Read the model definition and answer for the solid it produces. Units are mm, in the model's axes. Coordinates: 2 decimals unless noted, no trailing zeros. Write each loop counter-clockwise with the first axis right and the second up, starting at its lowest first coordinate (ties: lowest second). Pieces come first, ordered by that corner, then holes.
(1) The part is cut by section B-B, the plane z = 2.25. Determine the outline of the cut face in (x, y).
(2) The part is cut by section A-A, the plane y = 3.8. Determine the outline of the cut face in (x, z), and give its area (3 significant figures).
(3) Straight lines are drawn through the part: line 1 along X through (y, z) = (4.6, 2); line 2 along Z through (x, y) = (9, 0.6). For each, find the intervals that lie inside material, in ascending order.
(4) The part is cut by section C-C, the plane x = 10. Determine the outline of the cut face in (y, z), and give its area (3 significant figures).
```python
from build123d import *

# Parameters (mm, degrees)
BOSS_EXTRUDE1_DEPTH = 5


with BuildPart() as part:
    # Sketch1 → Boss-Extrude1 (new body)
    with BuildSketch(Plane(origin=(0, 0, 0), x_dir=(1, 0, 0), z_dir=(0, 1, 0))):
        with BuildLine():
            Line((75, -15), (75, 0))
            Line((75, 0), (14.1, 0))
            ThreePointArc((14.1, 0), (10, -4.1), (5.9, 0))
            Line((5.9, 0), (0, 0))
            Line((0, 0), (0, -15))
            Line((0, -15), (75, -15))
        make_face()
        with BuildLine():
            Line((135.9, 0), (75, 0))
            Line((75, 0), (75, -15))
            Line((75, -15), (150, -15))
            Line((150, -15), (150, 0))
            Line((150, 0), (144.1, 0))
            ThreePointArc((144.1, 0), (140, -4.1), (135.9, 0))
        make_face()
    extrude(amount=BOSS_EXTRUDE1_DEPTH)


solid = part.part
```
Computed:
1. outline: (0, 0) - (6.57, 0) - (6.57, 5) - (0, 5) - close; (13.43, 0) - (136.57, 0) - (136.57, 5) - (13.43, 5) - close; (143.43, 0) - (150, 0) - (150, 5) - (143.43, 5) - close
2. outline: (0, 0) - (5.9, 0) arc R4.1 cw to (14.1, 0) - (135.9, 0) arc R4.1 cw to (144.1, 0) - (150, 0) - (150, 15) - (0, 15) - close
2. area: 2,200 mm2
3. line 1: x = 0 to 6.42, 13.58 to 136.42, 143.58 to 150
3. line 2: z = 3.98 to 15
4. outline: (0, 4.1) - (5, 4.1) - (5, 15) - (0, 15) - close
4. area: 54.5 mm2
